Build history of the part. All positions in model axes, mm. Coordinates: 2 decimals unless noted, no trailing zeros. Loops run counter-clockwise (first coordinate to the right, second up) from the corner with the lowest first, then second, coordinate; pieces in that order, holes last.
Item 1: Cut at C-C (y = -4.25). List the corners of the cut face in (x, z).
Item 2: Cut at D-D (x = 18). List the corners of the cut face in (y, z).
Item 3: Cut at B-B (z = 7.25). List the corners of the cut face in (x, y), and give its area (3 significant figures).
Item 4: Mould opens along X. For faces 1 (the face through (2, -2, 10)), 2 (the face through (46.436, -0.17, 2.465)), 3 (the face through (-10, 0, 5)) say: released by +X, released by -X, zero draft, split by the parting line, or undercut.
Item 5: Cut at A-A (z = 1). List the corners of the cut face in (x, y).
Item 6: Flat gauge pins, fed straight in: pin 1 (3.5 mm diameter, centred on x = 45, y = -0.62, fed in from +Z); pin 2 (4 mm diameter, centred on y = 5, z = 3, fed in from +X). Where does each tip first touch, or does it go through?
Item 7: Drill centre lines: line 1 along Y through (x, z) = (0, 5.25); line 2 along X through (y, z) = (-2, 0.75); line 3 along Z through (x, y) = (31.5, -3.75). Where is each one in solid material? Low to high.
from build123d import *

# Parameters (mm, degrees)
SKETCH1_R           = 2.51
BOSS_EXTRUDE1_DEPTH = 10
SKETCH1_3_R         = 7.5
SKETCH1_3_R_2       = 1.51
BOSS_EXTRUDE2_DEPTH = 5


with BuildPart() as part:
    # Sketch1 → Boss-Extrude1 (new body)
    with BuildSketch(Plane.XY):
        with BuildLine():
            Line((1.373905706, 9.905169514), (0, 10))
            ThreePointArc((0, 10), (-10, 0), (0, -10))
            Line((0, -10), (0.829742277, -9.965516934))
            ThreePointArc((0.829742277, -9.965516934), (7.3585808, -6.771357959), (10, 0))
            ThreePointArc((10, 0), (7.541188801, 6.567379346), (1.373905706, 9.905169514))
        make_face()
        Circle(SKETCH1_R, mode=Mode.SUBTRACT)
    extrude(amount=BOSS_EXTRUDE1_DEPTH)

    # Sketch1_3 → Boss-Extrude2 (add)
    # profile 1 of 2: a face of its own
    with BuildSketch(Plane.XY):
        with BuildLine():
            Line((45.512119929, 6.858637088), (1.373905706, 9.905169514))
            ThreePointArc((1.373905706, 9.905169514), (7.541188801, 6.567379346), (10, 0))
            ThreePointArc((10, 0), (7.3585808, -6.771357959), (0.829742277, -9.965516934))
            Line((0.829742277, -9.965516934), (45.307101416, -8.117092704))
            ThreePointArc((45.307101416, -8.117092704), (37.496382194, -0.520895302), (45.512119929, 6.858637088))
        make_face()
    # profile 2 of 2: a face of its own
    with BuildSketch(Plane.XY):
        with Locations((44.995679477, -0.623561069)):
            Circle(SKETCH1_3_R)
        with Locations((44.995679477, -0.623561069)):
            Circle(SKETCH1_3_R_2, mode=Mode.SUBTRACT)
    extrude(amount=BOSS_EXTRUDE2_DEPTH)


solid = part.part
Filled sheet:
1. outline: (-9.05, 0) - (51.56, 0) - (51.56, 5) - (9.05, 5) - (9.05, 10) - (-9.05, 10) - close
2. outline: (-9.25, 0) - (8.76, 0) - (8.76, 5) - (-9.25, 5) - close
3. outline: (0, -10) - (0.83, -9.97) arc R10 ccw to (1.37, 9.91) - (0, 10) arc R10 ccw to start; hole circle Ø5.02 at (0, 0)
3. area: 294 mm2
4. face 1: zero draft
4. face 2: undercut
4. face 3: released by -X
5. outline: (0, -10) - (45.31, -8.12) arc R7.5 ccw to (45.51, 6.86) - (0, 10) arc R10 ccw to start; hole circle Ø5.02 at (0, 0); hole circle Ø3.02 at (45, -0.62)
6. pin 1: stops at z = 5
6. pin 2: stops at x = 51.56
7. line 1: y = -10 to -2.51, 2.51 to 10
7. line 2: x = -9.8 to -1.52, 1.52 to 44.37, 45.62 to 52.37
7. line 3: z = 0 to 5
